Autodesk Inventor part; units mm, degrees
ref_plane "YZ Plane" through (0, 0, 0) normal (1, 0, 0) x (0, 1, 0)
ref_plane "XZ Plane" through (0, 0, 0) normal (0, 1, 0) x (-1, 0, 0)
ref_plane "XY Plane" through (0, 0, 0) normal (0, 0, 1) x (1, 0, 0)
sketch "Sketch_1" plane through (0, 0, 0) normal (0, 0, 1) x (1, 0, 0)
  line L0 (63.5, 0) -> (0, 0)
  line L1 (0, 0) -> (0, 2)
  line L2 (0, 2) -> (0.5, 2.5)
  line L3 (0.5, 2.5) -> (63, 2.5)
  line L4 (63, 2.5) -> (63.5, 2)
  line L5 (63.5, 2) -> (63.5, 0)
  line L6 (63.5, 0) -> (0, 0)
revolve "Revolution1" add sketch "Sketch_1" angle 360 about axis through (63.5, 0, 0) along (1, 0, 0)
sketch "Sketch2" plane through (0, 0, 0) normal (-1, 0, 0) x (0, 0, 1)
  point P0 (0, 0)
hole "Hole1" at (0, 0, 0) direction (1, 0, 0) diameter 2.459 depth 8.2901 tip angle 120 countersink diameter 3 countersink angle 90
sketch "Sketch3" plane through (63.5, 0, 0) normal (1, 0, 0) x (0, 0, -1)
  point P0 (0, 0)
hole "Hole2" at (63.5, 0, 0) direction (-1, 0, 0) diameter 2.459 depth 8.2901 tip angle 120 countersink diameter 3 countersink angle 90
properties part number "SETF5-63.5-M3-N3" material "ステンレス鋼 AISI 304"
Here's how the part is built. I have some questions about the finished solid (model axes, mm). A direction names the side the tool comes from. Give positions to 0.01 mm unless a question says otherwise; leave off trailing zeros. Loops run counter-clockwise (first coordinate to the right, second up) from the corner with the lowest first, then second, coordinate; pieces in that order, holes last. Notation, with made-up numbers: M 53.5,40.5 L 76.5,40.5 A17 cw 76.5,47.5 Z; hole C -4,53.25 d9. An arc over 180 degrees is marked long. Put each result on its own line as item: value. Start each with the question number.
(1) For faces 1 (the cylindrical face through (59.164, 0.748, 0.976)), 2 (the cylindrical face through (4.336, 0.748, -0.976)), which set-ups out of +Z, -Z, +X, -X, +Y, -Y let a thin tool reach every point of the face, with its end or its side?
(2) I need wall thicknesses on line 1 along Z through (x, y) = (5.5, 0); line 2 along Y through (x, z) = (3.5, 1.4); line 3 along Z through (x, y) = (49, 0.15). Which ranges of each line are inside material? Lowest first, please. Write a range as [from, to].
(3) If we mould it in two halves opening along Z, with no side actions, what happens to faces 3 (the conical face through (54.62, 0.06, -0.2)), 4 (the cylindrical face through (32.19, -0.54, -2.44))? For each: +Z half, -Z half, draft (parallel to the pull), parting line (faces both ways), or undercut.
(4) Will these pins go through, and if not, where does the flat tip stop? pin 1 Ø2 at (y, z) = (0, 0) entering from +X; pin 2 Ø2 at (x, z) = (39, 2) entering from +Y; pin 3 Ø1.5 at (x, z) = (21.5, -1.5) entering from -Y.
(5) I want a section at A-A on x = 11.5. Please give me the cut outline in (y, z), then the cut area to 3 significant figures.
Answer block:
1. face 1: +X
1. face 2: -X
2. line 1: [-2.5, -1.23], [1.23, 2.5]
2. line 2: [-2.07, 2.07]
2. line 3: [-2.5, 2.5]
3. face 3: undercut
3. face 4: parting line
4. pin 1: x = 55.08
4. pin 2: y = 2.29
4. pin 3: y = -2.38
5. outline: C 0,0 d5
5. area: 19.6 mm^2
